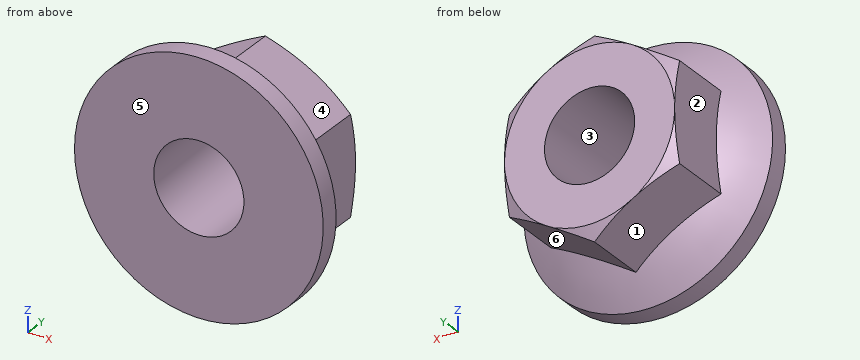
from build123d import *

# Parameters (mm, degrees)
BOSS_EXTRUDE1_DEPTH = 5
TAP1_D              = 4.134


with BuildPart() as part:
    # Sketch1 → Revolve1 (revolve)
    with BuildSketch(Plane.XY):
        with BuildLine():
            Line((0, 0), (-5.7, 0))
            Line((-5.7, 0), (-5.7, 0.9))
            ThreePointArc((-5.7, 0.9), (-3.03726851, 2.458300241), (0, 3))
            Line((0, 3), (0, 0))
        make_face()
    revolve(axis=Axis((0, 55, 0), (0, -1, 0)))

    # Sketch2 → Boss-Extrude1 (add)
    with BuildSketch(Plane.XZ):
        Polygon((0, 4.5033321), (-3.9, 2.25166605), (-3.9, -2.25166605), (0, -4.5033321), (3.9, -2.25166605), (3.9, 2.25166605), align=None)
    extrude(amount=-BOSS_EXTRUDE1_DEPTH)

    # Sketch3 → Cut-Revolve1 (revolve, cut)
    with BuildSketch(Plane.XY):
        Polygon((-3.9, 5), (-5.9, 5), (-5.9, 3.845299462), align=None)
    revolve(axis=Axis((0, 55, 0), (0, -1, 0)), mode=Mode.SUBTRACT)

    # Tap1 (through all)
    with Locations(Plane(origin=(0, 5, 0), x_dir=(1, 0, 0), z_dir=(0, 1, 0))):
        with Locations((0, 0)):
            Hole(TAP1_D / 2)


solid = part.part
Source: CAD feature listing. Evaluate the final solid. Frame: model axes, mm. Face numbers are marked on the shaded views. A direction names the side the tool comes from. Give positions to 0.01 mm unless a question says otherwise; leave off trailing zeros. Write each loop counter-clockwise with the first axis right and the second up, starting at its lowest first coordinate (ties: lowest second). Pieces come first, ordered by that corner, then holes. Notation, with made-up numbers: (17, 10.25) - (63, 10.25) arc R16 ccw to (63, 31.25) - close; hole circle Ø11 at (61.25, 34.25). An arc over 180 degrees is marked (long way). Write item = value, one per line. Start each with the question number.
Q1. Draft query along Z for the marked faces 1, 2, 3 and 4. Return one class per face: +Z half, -Z half, draft (parallel to the pull), parting line (faces both ways), or undercut.
Q2. Material intervals for probe 1 along X at (y, z) = (3.6, -1); probe 2 along Z at (x, y) = (-1, 3.35); probe 3 along Z at (x, y) = (1.5, 2.25), sorted ascending.
Q3. Cut plane C-C, the plane y = 0.45. Return loops of the section in (x, z), then the cut area to 3 significant figures.
Q4. Reachability of the marked faces 5 and 6 from +Z, -Z, +X, -X, +Y, -Y: full face, straight path, thin tool, end or side. Return the list, or none.
Q5. Cut plane A-A, the plane y = 2.75. Return loops of the section in (x, z), then the cut area to 3 significant figures.
Q6. Cut plane B-B, the plane x = -4.5. Return loops of the section in (y, z), then the cut area to 3 significant figures.
Q7. Pin query (flat end, axial travel): pin 1 Ø6.5 at (x, z) = (0, 0) entering from +Y; pin 2 Ø3 at (y, z) = (2.5, 0) entering from +X; pin 3 Ø1 at (y, z) = (3.5, 0.5) entering from -X; pin 4 Ø3 at (y, z) = (4, -1) entering from +X. Return the tip coordinate at first contact, or that it passes through.
Q8. Cut plane D-D, the plane x = 4.75. Return loops of the section in (y, z).
Computed values:
q1.face_1 = -Z half
q1.face_2 = draft
q1.face_3 = undercut
q1.face_4 = +Z half
q2.probe_1 = -3.9 to -1.81, 1.81 to 3.9
q2.probe_2 = -3.93 to -1.81, 1.81 to 3.93
q2.probe_3 = -3.64 to -1.42, 1.42 to 3.64
q3.outline = circle Ø11.4 at (0, 0); hole circle Ø4.13 at (0, 0)
q3.area = 88.6 mm²
q4.face_5 = +Z, -Z, +X, -X, -Y
q4.face_6 = -Z, +X, +Y
q5.outline = (-3.9, -2.25) - (0, -4.5) - (3.9, -2.25) - (3.9, 2.25) - (0, 4.5) - (-3.9, 2.25) - close; hole circle Ø4.13 at (0, 0)
q5.area = 39.3 mm²
q6.outline = (0, -3.5) - (0.9, -3.5) arc R7.55 ccw to (0.9, 3.5) - (0, 3.5) - close
q6.area = 10.4 mm²
q7.pin_1 = 5
q7.pin_2 = 5.58
q7.pin_3 = -3.9
q7.pin_4 = 3.9
q8.outline = (0, -3.15) - (0.9, -3.15) arc R7.39 ccw to (0.9, 3.15) - (0, 3.15) - close
